For this review, use the dimensioned drawing (mm, ordinates from the lowest corner) and the shaded views. A direction names the side the tool comes from. Coordinates: 2 decimals unless noted, no trailing zeros. Write each loop counter-clockwise with the first axis right and the second up, starting at its lowest first coordinate (ties: lowest second). Pieces come first, ordered by that corner, then holes. Notation, with made-up numbers: M 61,10 L 84,10 A9 ccw 84,22 Z; hole C -27.5,-38.75 d6. An arc over 180 degrees is marked long. Return JSON: item names as keys, results as strings. Group by question number.
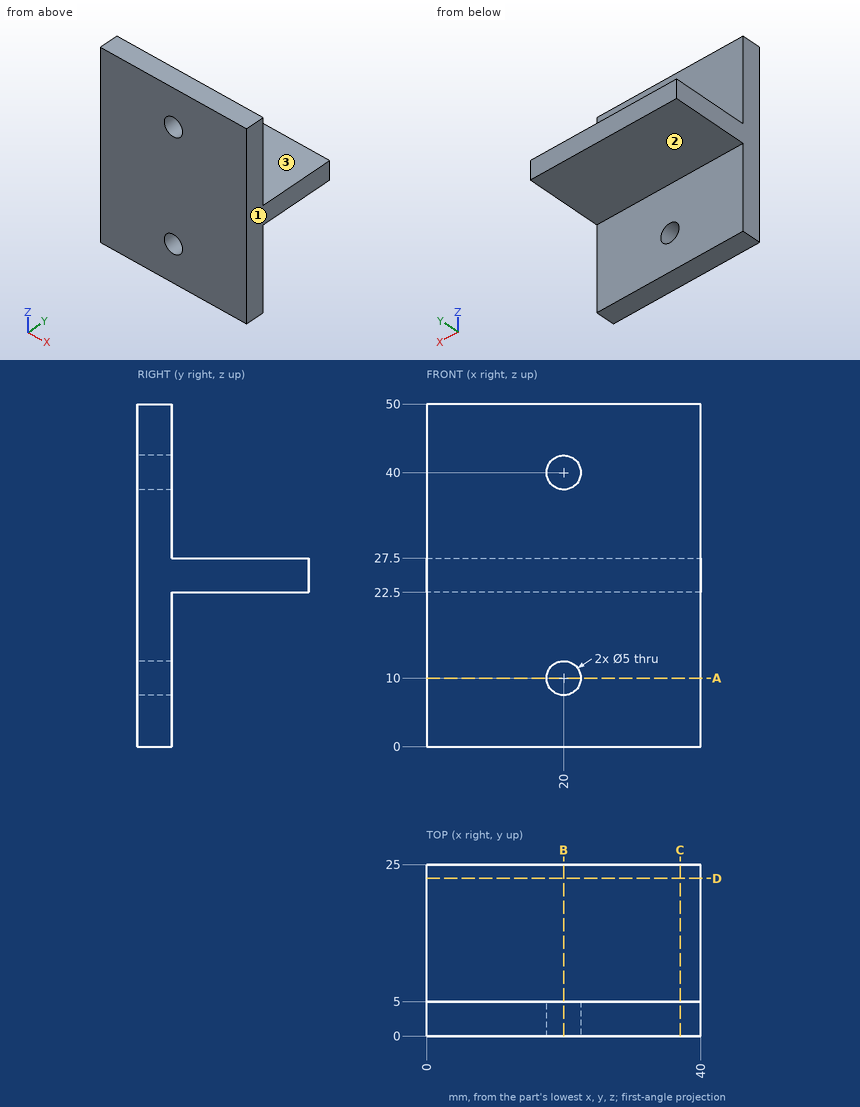
Item 1: Add section D-D (y = 23). Write out the cut boundary in (x, z), plus the area to 3 significant figures.
Item 2: Add section C-C (x = 37). Write out the cut boundary in (y, z).
Item 3: For pin 1 (11 mm diameter, centred on x = 12, z = 8.5, fed in from +Y); pin 2 (1.5 mm diameter, centred on x = 10.5, y = 11.5, fed in from -Z); pin 3 (8 mm diameter, centred on x = 20, z = 10, fed in from -Y), all flat-tipped, find the tip position at first contact; note any pin that passes through.
Item 4: Machinability: for the marked faces 1, 2 and 3, which of the approach directions +Z, -Z, +X, -X, +Y, -Y give a long, thin tool a straight path to every point of the face, cutting with its end or side? Answer none if there is none.
Item 5: Add section A-A (z = 10). Write out the cut boundary in (x, y).
Item 6: For line 1 (Z direction, x = 20, y = 1.35); line 2 (Z direction, x = 34, y = 18.5); line 3 (Y direction, x = 29, z = 41.5), list the stretches that pass through material, from the lowest coordinate up.
Item 7: Add section B-B (x = 20). Write out the cut boundary in (y, z).
Geometry check:
{
 "1": {"outline": "M 0,22.5 L 40,22.5 L 40,27.5 L 0,27.5 Z", "area": "200 mm^2"},
 "2": {"outline": "M 0,0 L 5,0 L 5,22.5 L 25,22.5 L 25,27.5 L 5,27.5 L 5,50 L 0,50 Z"},
 "3": {"pin 1": "y = 5", "pin 2": "z = 22.5", "pin 3": "y = 0"},
 "4": {"face 1": "+Z, -Z, +X, +Y, -Y", "face 2": "-Z, +X, -X, +Y", "face 3": "+Z, +X, -X, +Y"},
 "5": {"outline": "M 0,0 L 17.5,0 L 17.5,5 L 0,5 Z; M 22.5,0 L 40,0 L 40,5 L 22.5,5 Z"},
 "6": {"line 1": "0 to 7.5, 12.5 to 37.5, 42.5 to 50", "line 2": "22.5 to 27.5", "line 3": "0 to 5"},
 "7": {"outline": "M 0,0 L 5,0 L 5,7.5 L 0,7.5 Z; M 0,12.5 L 5,12.5 L 5,22.5 L 25,22.5 L 25,27.5 L 5,27.5 L 5,37.5 L 0,37.5 Z; M 0,42.5 L 5,42.5 L 5,50 L 0,50 Z"}
}
